```python
from build123d import *

# Parameters (mm, degrees)
SKETCH1_W               = 920
SKETCH1_H               = 40
BOSS_EXTRUDE1_DEPTH     = 40
FILLET1_R               = 3
SHELL1_START            = -497
SHELL1_OUTLINE_W        = 34
SHELL1_OUTLINE_H        = 34
SHELL1_DEPTH            = 994
SHELL1_2_OUTLINE_W      = 626
SHELL1_2_OUTLINE_H      = 34
SHELL1_2_OUTLINE_W_2    = 785
SHELL1_2_DEPTH          = 34
SHELL1_START_2          = 463
SHELL1_3_OUTLINE_W      = 626
SHELL1_3_OUTLINE_H      = 34
SHELL1_3_OUTLINE_W_2    = 785
SHELL1_3_DEPTH          = 34
SKETCH4_R               = 9
CUT_EXTRUDE2_DEPTH      = 1492.852874784
SKETCH5_W               = 34
SKETCH5_H               = 34
CUT_EXTRUDE3_DEPTH      = 1565.749181179
CUT_EXTRUDE4_DEPTH      = 966.7851728
CUT_EXTRUDE4_DEPTH_BACK = 966.7851728
SKETCH6_R               = 5


# Read off the part's stored shape, not the designer's step: Shell1
with BuildPart() as part:
    # Sketch1 → Boss-Extrude1 (new body)
    with BuildSketch(Plane.XY.offset(6)):
        Polygon((500, -1405), (460, -1405), (460, 40), (-460, 40), (-460, -1405), (-500, -1405), (-500, 80), (500, 80), align=None)
        with Locations((0, -600)):
            Rectangle(SKETCH1_W, SKETCH1_H)
        Polygon((-460, -1405), (-460, 40), (-500, 80), (-500, -1405), align=None)
        Polygon((-460, 40), (460, 40), (500, 80), (-500, 80), align=None)
    extrude(amount=BOSS_EXTRUDE1_DEPTH)

    # Fillet1
    fillet1_edges = [part.edges().sort_by_distance(p)[0] for p in [
        (0, 40, 6),
        (460, -270, 6),
        (0, -580, 6),
        (-500, -662.5, 6),
        (-460, -1012.5, 6),
        (0, -620, 6),
        (460, -1012.5, 6),
        (500, -662.5, 6),
        (500, 80, 26),
        (-500, 80, 26),
        (0, 80, 6),
        (0, -580, 46),
        (460, -270, 46),
        (0, 40, 46),
        (-460, -270, 46),
        (500, -662.5, 46),
        (460, -1012.5, 46),
        (0, -620, 46),
        (-460, -1012.5, 46),
        (-500, -662.5, 46),
        (0, 80, 46),
    ]]
    fillet(fillet1_edges, radius=FILLET1_R)

    # Shell1 outline → Shell1 (cut)
    with BuildSketch(Plane.YZ.offset(SHELL1_START)):
        with Locations((60, 26)):
            Rectangle(SHELL1_OUTLINE_W, SHELL1_OUTLINE_H)
        with Locations((-600, 26)):
            Rectangle(SHELL1_OUTLINE_W, SHELL1_OUTLINE_H)
    extrude(amount=SHELL1_DEPTH, mode=Mode.SUBTRACT)

    # Shell1 2 outline → Shell1 2 (cut)
    with BuildSketch(Plane.YZ.offset(SHELL1_START)):
        with Locations((-270, 26)):
            Rectangle(SHELL1_2_OUTLINE_W, SHELL1_2_OUTLINE_H)
        with Locations((-1009.5, 26)):
            Rectangle(SHELL1_2_OUTLINE_W_2, SHELL1_2_OUTLINE_H)
    extrude(amount=SHELL1_2_DEPTH, mode=Mode.SUBTRACT)

    # Shell1 3 outline → Shell1 3 (cut)
    with BuildSketch(Plane.YZ.offset(SHELL1_START_2)):
        with Locations((-270, 26)):
            Rectangle(SHELL1_3_OUTLINE_W, SHELL1_3_OUTLINE_H)
        with Locations((-1009.5, 26)):
            Rectangle(SHELL1_3_OUTLINE_W_2, SHELL1_3_OUTLINE_H)
    extrude(amount=SHELL1_3_DEPTH, mode=Mode.SUBTRACT)

    # Sketch4 → Cut-Extrude2 (cut, through all)
    with BuildSketch(Plane.XY.offset(46)):
        with Locations((-350, 60)):
            Circle(SKETCH4_R)
        with Locations((0, 60)):
            Circle(SKETCH4_R)
        with Locations((350, 60)):
            Circle(SKETCH4_R)
    extrude(amount=-CUT_EXTRUDE2_DEPTH, mode=Mode.SUBTRACT)

    # Sketch5 → Cut-Extrude3 (cut, through all)
    with BuildSketch(Plane(origin=(0, -1402, 0), x_dir=(1, 0, 0), z_dir=(0, 1, 0))):
        with Locations((480, -26)):
            Rectangle(SKETCH5_W, SKETCH5_H)
        with Locations((-480, -26)):
            Rectangle(SKETCH5_W, SKETCH5_H)
    extrude(amount=-CUT_EXTRUDE3_DEPTH, mode=Mode.SUBTRACT)

    # Sketch6 → Cut-Extrude4 (cut, two sides: drawn at the far end of the back side and taken through both)
    with BuildSketch(Plane(origin=(0, -580, 0), x_dir=(1, 0, 0), z_dir=(0, 1, 0)).offset(-CUT_EXTRUDE4_DEPTH_BACK)):
        with Locations(Location((-387.5, -26, 0), (0, 0, 270))):
            Circle(SKETCH6_R)
        with Locations(Location((-312.5, -26, 0), (0, 0, 270))):
            Circle(SKETCH6_R)
        with Locations(Location((312.5, -26, 0), (0, 0, 270))):
            Circle(SKETCH6_R)
        with Locations(Location((387.5, -26, 0), (0, 0, 270))):
            Circle(SKETCH6_R)
    extrude(amount=CUT_EXTRUDE4_DEPTH + CUT_EXTRUDE4_DEPTH_BACK, mode=Mode.SUBTRACT)


solid = part.part
```
Can you work these out from the model? Positions are in its coordinate system, mm. A direction names the side the tool comes from. Give positions to 0.01 mm unless a question says otherwise; leave off trailing zeros. Loops run counter-clockwise (first coordinate to the right, second up) from the corner with the lowest first, then second, coordinate; pieces in that order, holes last. Notation, with made-up numbers: M 48.25,-21.75 L 64.25,-21.75 A13 ccw 64.25,2.25 Z; hole C 20.5,19.25 d8. An arc over 180 degrees is marked long. Use CSV: the item, a comma, the result in double quotes. Start each with the question number.
1. If we mould it in two halves opening along X, with no side actions, what happens to faces 4 (the face through (500, -654, 26)), 5 (the face through (462.5, -1405, 25.7)), 6 (the face through (-6, -580, 26))? For each: released by +X, released by -X, zero draft, split by the parting line, or undercut.
2. Imagine slicing it at A-A, the plane y = -240. Write out the boundary of the cut face in (x, z).
3. Imagine slicing it at C-C, the plane y = -915.5. Write out the boundary of the cut face in (x, z).
4. Imagine slicing it at B-B, the plane x = 188. Write out the boundary of the cut face in (y, z), plus the area to 3 significant figures.
5. For P1, Ø17, axis at x = 123, z = 33.5, coming from the -Y side; P2, Ø20.5, axis at x = 0, y = 60, coming from the -Z side, each with a flat end and sliding along its axis, tell me the tip position at first contact or that it passes through.
6. If I drill on L1, parallel to X at y = -389, z = 38; L2, parallel to Y at x = 178, z = 42; L3, parallel to Y at x = -350, z = 44, over which ranges is the centre line in solid material (lowest first)?
7. On a 3-axis mill with a long thin cutter (end or side, diameter ignored), from which of +Z, -Z, +X, -X, +Y, -Y can I reach the whole of each face in a straight line? I mean faces 1 (the face through (460, -1018, 26)), 2 (the face through (-460, -266, 24)), 3 (the face through (-463, -274, 26)). Say none if no direction works.
Response values:
1,face 4,"released by +X"
1,face 5,"zero draft"
1,face 6,"undercut"
2,outline,"M -500,9 A3 ccw -497,6 L -460,6 L -460,43 A3 ccw -463,46 L -497,46 A3 ccw -500,43 Z; M 460,9 A3 ccw 463,6 L 497,6 A3 ccw 500,9 L 500,43 A3 ccw 497,46 L 463,46 A3 ccw 460,43 Z; hole M -497,9 L -463,9 L -463,43 L -497,43 Z; hole M 463,9 L 497,9 L 497,43 L 463,43 Z"
3,outline,"M -500,9 A3 ccw -497,6 L -463,6 A3 ccw -460,9 L -460,43 A3 ccw -463,46 L -497,46 A3 ccw -500,43 Z; M 460,9 A3 ccw 463,6 L 497,6 A3 ccw 500,9 L 500,43 A3 ccw 497,46 L 463,46 A3 ccw 460,43 Z; hole M -497,9 L -463,9 L -463,43 L -497,43 Z; hole M 463,9 L 497,9 L 497,43 L 463,43 Z"
4,outline,"M -620,9 A3 ccw -617,6 L -583,6 A3 ccw -580,9 L -580,43 A3 ccw -583,46 L -617,46 A3 ccw -620,43 Z; M 40,9 A3 ccw 43,6 L 77,6 A3 ccw 80,9 L 80,43 A3 ccw 77,46 L 43,46 A3 ccw 40,43 Z; hole M -617,9 L -583,9 L -583,43 L -617,43 Z; hole M 43,9 L 77,9 L 77,43 L 43,43 Z"
4,area,"873 mm^2"
5,P1,"y = -620"
5,P2,"z = 6"
6,L1,"-500 to -497, -463 to -460, 460 to 463, 497 to 500"
6,L2,"-620 to -617, -583 to -580, 40 to 43, 77 to 80"
6,L3,"-619.83 to -580.17, 40.17 to 51, 69 to 79.83"
7,face 1,"+Z, -Z, -Y"
7,face 2,"+Z, -Z"
7,face 3,"-Y"
